Check sheet for the modelled part. Datum: model origin and axes. Units: mm. Face numbers are marked on the shaded views. A direction names the side the tool comes from. Round coordinates to 2 decimals unless told otherwise and drop trailing zeros. Write each loop counter-clockwise with the first axis right and the second up, starting at its lowest first coordinate (ties: lowest second). Pieces come first, ordered by that corner, then holes. Notation, with made-up numbers: M 2.5,62 L 55.5,62 A19 cw 55.5,72 Z; hole C 70.5,13 d2. An arc over 180 degrees is marked long. Answer in a Markdown table with one row per item.
```python
from build123d import *

# Parameters (mm, degrees)
SKETCH1_R           = 34.925
SKETCH1_R_2         = 19.05
BOSS_EXTRUDE1_DEPTH = 85.725
BOSS_EXTRUDE2_DEPTH = 53.975
SKETCH1_4_W         = 57.15
SKETCH1_4_H         = 28.575
BOSS_EXTRUDE3_DEPTH = 22.225
BOSS_EXTRUDE4_DEPTH = 15.875
FILLET1_SIZE        = 19.05
SKETCH2_R           = 7.9375
CUT_EXTRUDE1_DEPTH  = 137.118289601


with BuildPart() as part:
    # Sketch1 → Boss-Extrude1 (new body)
    with BuildSketch(Plane(origin=(0, 0, 0), x_dir=(0, 0, -1), z_dir=(1, 0, 0))):
        Circle(SKETCH1_R)
        Circle(SKETCH1_R_2, mode=Mode.SUBTRACT)
    extrude(amount=BOSS_EXTRUDE1_DEPTH)

    # Sketch1<3> → Boss-Extrude2 (add)
    with BuildSketch(Plane(origin=(0, 0, 0), x_dir=(0, 0, -1), z_dir=(1, 0, 0))):
        with BuildLine():
            Line((69.85, 44.45), (12.7, 44.45))
            Line((12.7, 44.45), (12.7, 32.534068682))
            ThreePointArc((12.7, 32.534068682), (20.479669269, 28.290259306), (26.940768363, 22.225))
            Line((26.940768363, 22.225), (69.85, 22.225))
            Line((69.85, 22.225), (69.85, 44.45))
        make_face()
    extrude(amount=BOSS_EXTRUDE2_DEPTH)

    # Sketch1<4> → Boss-Extrude3 (add)
    with BuildSketch(Plane(origin=(0, 0, 0), x_dir=(0, 0, -1), z_dir=(1, 0, 0))):
        with Locations((41.275, 58.7375)):
            Rectangle(SKETCH1_4_W, SKETCH1_4_H)
    extrude(amount=BOSS_EXTRUDE3_DEPTH)

    # Sketch1<5> → Boss-Extrude4 (add)
    with BuildSketch(Plane(origin=(0, 0, 0), x_dir=(0, 0, -1), z_dir=(1, 0, 0))):
        with BuildLine():
            Line((12.7, 32.534068682), (12.7, 44.45))
            Line((12.7, 44.45), (12.7, 73.025))
            ThreePointArc((12.7, 73.025), (-22.035822369, 43.636405893), (-34.925, 0))
            ThreePointArc((-34.925, 0), (-19.700356913, 28.838369623), (12.7, 32.534068682))
        make_face()
    extrude(amount=BOSS_EXTRUDE4_DEPTH)

    # Fillet1
    # a fillet whose section is not a circle: 19.05 mm, written as the material it takes off along each edge
    with BuildSketch(Plane(origin=(53.975, -25.4, -69.85), x_dir=(0, 0, 1), z_dir=(0, 1, 0))) as fillet1_piece_1:
        with BuildLine():
            Bezier((FILLET1_SIZE, 0), (0, 0), (0, -FILLET1_SIZE), weights=[1, 1, 1])
            Line((0, -FILLET1_SIZE), (0, 0))
            Line((0, 0), (FILLET1_SIZE, 0))
        make_face()
    extrude(amount=117.475, mode=Mode.SUBTRACT)

    # Sketch2 → Cut-Extrude1 (cut, through all)
    with BuildSketch(Plane(origin=(0, 44.45, 0), x_dir=(1, 0, 0), z_dir=(0, 1, 0))):
        with Locations(Location((34.925, 50.8, 0), (0, 0, 270))):
            Circle(SKETCH2_R)
    extrude(amount=-CUT_EXTRUDE1_DEPTH, mode=Mode.SUBTRACT)


solid = part.part
```
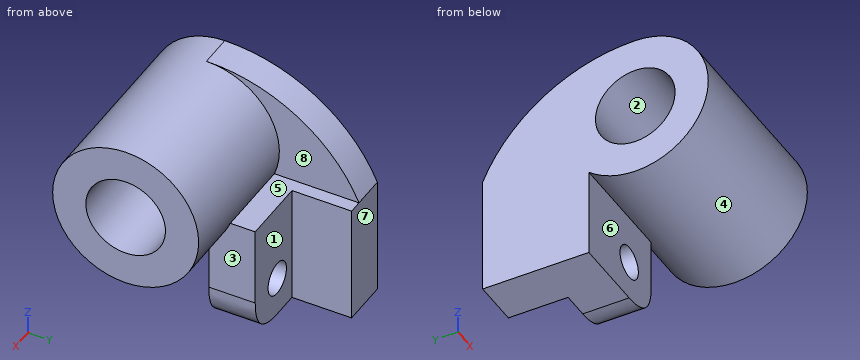
1. Section check D-D, the plane x = 6. Record the cut outline in (y, z) (3 decimals).
Found:
| item | result |
|---|---|
| outline | M 0,34.925 A34.925 ccw long 22.225,-26.941 L 22.225,-69.85 L 73.025,-69.85 L 73.025,-12.7 A79.375 ccw Z; hole C 0,0 d38.1 |
2. Section check B-B, the plane x = 32. Record the cut outline in (y, z) (3 decimals).
Found:
| item | result |
|---|---|
| outline | M 22.225,-69.85 L 44.45,-69.85 L 44.45,-58.179 L 22.225,-58.179 Z; M 22.225,-43.421 L 44.45,-43.421 L 44.45,-12.7 L 32.534,-12.7 A34.925 ccw long 22.225,-26.941 Z; hole C 0,0 d38.1 |
3. Section check C-C, the plane y = -10. Record the cut outline in (x, z) (3 decimals), and give its area (3 significant figures).
Found:
| item | result |
|---|---|
| outline | M 0,-33.463 L 85.725,-33.463 L 85.725,-16.214 L 0,-16.214 Z; M 0,16.214 L 85.725,16.214 L 85.725,33.463 L 0,33.463 Z |
| area | 2,960 mm2 |
4. Go/stop test with flat-tipped pins: pin 1 (5 mm diameter, centred on y = 42.5, z = -26.5, fed in from -X); pin 2 (5 mm diameter, centred on x = 66.5, y = -11, fed in from +Z); pin 3 (1 mm diameter, centred on y = 32, z = -50.5, fed in from +X) (3 decimals); pin 4 (12 mm diameter, centred on y = 43.5, z = -4, fed in from +X) (3 decimals). Record where each tip stops, or that it passes through.
Found:
| item | result |
|---|---|
| pin 1 | stops at x = 0 |
| pin 2 | stops at z = 33.87 |
| pin 3 | stops at x = 53.975 |
| pin 4 | stops at x = 15.875 |
5. Section check A-A, the plane z = 13. Record the cut outline in (x, y) (3 decimals).
Found:
| item | result |
|---|---|
| outline | M 0,-32.415 L 85.725,-32.415 L 85.725,-13.925 L 0,-13.925 Z; M 0,13.925 L 85.725,13.925 L 85.725,32.415 L 15.875,32.415 L 15.875,55.048 L 0,55.048 Z |
6. Access from +Z, -Z, +X, -X, +Y, -Y to the whole of each face (thin tool, end or side, straight path). Record for the marked faces 1, 2, 3, 4 and 5.
Found:
| item | result |
|---|---|
| face 1 | +Z, -Z, +X, +Y |
| face 2 | +X, -X |
| face 3 | -Z, +X, +Y |
| face 4 | +X |
| face 5 | +X, +Y |
7. Draft check along Y on the marked faces 6, 7 and 8. Enter one of: +Y half, -Y half, draft (parallel to the pull), parting line (faces both ways), or undercut.
Found:
| item | result |
|---|---|
| face 6 | undercut |
| face 7 | +Y half |
| face 8 | draft |
8. Scan lines: L1, parallel to X at y = 30.25, z = -50.8 (1 decimal); L2, parallel to Y at x = 18, z = -35 (3 decimals); L3, parallel to Y at x = 44.5, z = 0 (3 decimals). Record each from-to range of solid material in increasing order.
Found:
| item | result |
|---|---|
| L1 | x = 0 to 27, 42.9 to 54 |
| L2 | y = 22.225 to 73.025 |
| L3 | y = -34.925 to -19.05, 19.05 to 34.925 |
